Can you work these out from the model? Positions are in its coordinate system, mm. A direction names the side the tool comes from. Round coordinates to 2 decimals unless told otherwise and drop trailing zeros. Order: outer loops, then holes, each group sorted by start corner. A loop starts at its lowest first (then second) coordinate and runs counter-clockwise, first axis right, second up.
from build123d import *

# Parameters (mm, degrees)
SKETCH_1_R      = 2.1
EXTRUDE_1_DEPTH = 3
FILLET_2_R      = 5


with BuildPart() as part:
    # 草图1 → 凸台-拉伸1 (new body)
    with BuildSketch(Plane(origin=(0, 0, 0), x_dir=(0, 0, -1), z_dir=(1, 0, 0))):
        Polygon((10, -10), (30, -10), (30, -30), (10, -30), (-10, -30), (-10, 30), (10, 30), align=None)
        with Locations((0, 20)):
            Circle(SKETCH_1_R, mode=Mode.SUBTRACT)
        Circle(SKETCH_1_R, mode=Mode.SUBTRACT)
        with Locations((0, -20)):
            Circle(SKETCH_1_R, mode=Mode.SUBTRACT)
        with Locations((20, -20)):
            Circle(SKETCH_1_R, mode=Mode.SUBTRACT)
    extrude(amount=EXTRUDE_1_DEPTH)

    # 圆角2
    fillet_2_edges = [part.edges().sort_by_distance(p)[0] for p in [
        (1.5, -30, 10),
        (1.5, 30, 10),
        (1.5, 30, -10),
        (1.5, -10, -10),
        (1.5, -10, -30),
        (1.5, -30, -30),
    ]]
    fillet(fillet_2_edges, radius=FILLET_2_R)


solid = part.part
(1) If we mould it in two halves opening along Z, with no side actions, what happens to faces 1 (the face through (3, -6, -6)), 2 (the face through (2, -11, -28)), 3 (the face through (1.48, 21.77, -1.13))? For each: pulls with the +Z half, pulls with the -Z half, needs draft (parallel to the pull), parting line crosses it, or undercut.
(2) I want a section at B-B, the plane x = 2.15. List the corners of the cut face in (y, z) for me, plus the area to 3 significant figures.
(3) I want a section at A-A, the plane y = 20. List the corners of the cut face in (x, z) for me, plus the area to 3 significant figures.
(4) Please list where these lines run through material, in increasing order: probe 1 along Y at (x, z) = (1.9, 0); probe 2 along Y at (x, z) = (1.35, -25); probe 3 along Z at (x, y) = (2.3, -4).
(5) On a 3-axis mill with a long thin cutter (end or side, diameter ignored), from which of +Z, -Z, +X, -X, +Y, -Y can I reach the whole of each face in a straight line? I mean faces 4 (the face through (1, 10, -10)), 5 (the face through (1, -20, -30)). Say none if no direction works.
(6) I want a section at D-D, the plane z = -19.5. List the corners of the cut face in (x, y) for me.
(7) I want a section at C-C, the plane z = 0. List the corners of the cut face in (x, y) for me.
(8) I'm going to push a flat-ended pin straight in: pin 1 Ø0.9 at (x, y) = (1.5, 12.5) entering from -Z. Where does the tip first touch, or does it pass through?
Ans:
1. face 1: needs draft
1. face 2: pulls with the -Z half
1. face 3: undercut
2. outline: (-30, -25) arc R5 ccw to (-25, -30) - (-15, -30) arc R5 ccw to (-10, -25) - (-10, -15) arc R5 cw to (-5, -10) - (25, -10) arc R5 ccw to (30, -5) - (30, 5) arc R5 ccw to (25, 10) - (-25, 10) arc R5 ccw to (-30, 5) - close; hole circle Ø4.2 at (-20, -20); hole circle Ø4.2 at (-20, 0); hole circle Ø4.2 at (0, 0); hole circle Ø4.2 at (20, 0)
2. area: 1,520 mm2
3. outline: (0, -10) - (3, -10) - (3, -2.1) - (0, -2.1) - close; (0, 2.1) - (3, 2.1) - (3, 10) - (0, 10) - close
3. area: 47.4 mm2
4. probe 1: y = -30 to -22.1, -17.9 to -2.1, 2.1 to 17.9, 22.1 to 30
4. probe 2: y = -30 to -10
4. probe 3: z = -10 to 10
5. face 4: -Z, +X, -X, +Y
5. face 5: -Z, +X, -X, +Y, -Y
6. outline: (0, -30) - (3, -30) - (3, -22.04) - (0, -22.04) - close; (0, -17.96) - (3, -17.96) - (3, -10) - (0, -10) - close
7. outline: (0, -30) - (3, -30) - (3, -22.1) - (0, -22.1) - close; (0, -17.9) - (3, -17.9) - (3, -2.1) - (0, -2.1) - close; (0, 2.1) - (3, 2.1) - (3, 17.9) - (0, 17.9) - close; (0, 22.1) - (3, 22.1) - (3, 30) - (0, 30) - close
8. pin 1: stops at z = -10
